from build123d import *

# Parameters (mm, degrees)
BOSS_EXTRUDE1_DEPTH = 5.5
FILLET1_R           = 0.75
FILLET2_R           = 3
SKETCH2_R           = 6
CUT_EXTRUDE1_DEPTH  = 16.19429676984497


with BuildPart() as part:
    # Sketch1 → Boss-Extrude1 (new body)
    with BuildSketch(Plane(origin=(0, 0, 0), x_dir=(1, 0, 0), z_dir=(0, 1, 0))):
        Polygon((10.969655114602853, 0), (5.484827557301405, 9.499999999999982), (-5.48482755730147, 9.499999999999945), (-10.969655114602851, -7.66e-14), (-5.484827557301339, -9.50000000000002), (5.4848275573015375, -9.499999999999904), align=None)
    extrude(amount=BOSS_EXTRUDE1_DEPTH)

    # Fillet1
    fillet1_edges = [part.edges().sort_by_distance(p)[0] for p in [
        (-3.286e-14, 5.5, -9.499999999999964),
        (-8.227241335952161, 5.5, -4.749999999999934),
        (-8.227241335952096, 5.5, 4.750000000000048),
        (9.859e-14, 5.5, 9.499999999999961),
        (8.227241335952195, 5.5, 4.749999999999952),
        (8.22724133595213, 5.5, -4.749999999999991),
    ]]
    fillet(fillet1_edges, radius=FILLET1_R)

    # Fillet2
    # the kernel refuses this fillet: 3 mm, written as the material it takes off along each edge
    with BuildSketch(Plane(origin=(3.752776749732533, 5.5, -6.499999999999977), x_dir=(0.8660254037844382, 0, -0.500000000000001), z_dir=(0.500000000000001, 0, 0.8660254037844382))) as fillet2_piece_1:
        with BuildLine():
            CenterArc((2.25, -0.75), 0.75, 0, 90)
            Line((3, -0.75), (3, 0))
            Line((3, 0), (2.25, 0))
        make_face()
    revolve(axis=Axis((3.752776749732533, 5.5, -6.499999999999977), (0, 1, 0)), revolution_arc=60.000000000000135, mode=Mode.SUBTRACT)
    with BuildSketch(Plane(origin=(7.505553499465103, 5.5, 1.221e-14), x_dir=(0.8660254037844416, 0, 0.49999999999999495), z_dir=(-0.49999999999999495, 0, 0.8660254037844416))) as fillet2_piece_2:
        with BuildLine():
            CenterArc((2.25, -0.75), 0.75, 0, 90)
            Line((3, -0.75), (3, 0))
            Line((3, 0), (2.25, 0))
        make_face()
    revolve(axis=Axis((7.505553499465103, 5.5, 1.221e-14), (0, 1, 0)), revolution_arc=59.99999999999973, mode=Mode.SUBTRACT)
    with BuildSketch(Plane(origin=(-3.752776749732577, 5.5, -6.49999999999995), x_dir=(-3.4e-15, 0, -1), z_dir=(1, 0, -3.4e-15))) as fillet2_piece_3:
        with BuildLine():
            CenterArc((2.25, -0.75), 0.75, 0, 90)
            Line((3, -0.75), (3, 0))
            Line((3, 0), (2.25, 0))
        make_face()
    revolve(axis=Axis((-3.752776749732577, 5.5, -6.49999999999995), (0, 1, 0)), revolution_arc=60.00000000000015, mode=Mode.SUBTRACT)
    with BuildSketch(Plane(origin=(3.7527767497326376, 5.5, 6.499999999999923), x_dir=(1.053e-14, 0, 1), z_dir=(-1, 0, 1.053e-14))) as fillet2_piece_4:
        with BuildLine():
            CenterArc((2.25, -0.75), 0.75, 0, 90)
            Line((3, -0.75), (3, 0))
            Line((3, 0), (2.25, 0))
        make_face()
    revolve(axis=Axis((3.7527767497326376, 5.5, 6.499999999999923), (0, 1, 0)), revolution_arc=59.99999999999973, mode=Mode.SUBTRACT)
    with BuildSketch(Plane(origin=(-7.505553499465096, 5.5, 5.373e-14), x_dir=(-0.8660254037844417, 0, -0.49999999999999484), z_dir=(0.49999999999999484, 0, -0.8660254037844417))) as fillet2_piece_5:
        with BuildLine():
            CenterArc((2.25, -0.75), 0.75, 0, 90)
            Line((3, -0.75), (3, 0))
            Line((3, 0), (2.25, 0))
        make_face()
    revolve(axis=Axis((-7.505553499465096, 5.5, 5.373e-14), (0, 1, 0)), revolution_arc=60.00000000000011, mode=Mode.SUBTRACT)
    with BuildSketch(Plane(origin=(-3.752776749732488, 5.5, 6.500000000000002), x_dir=(-0.8660254037844347, 0, 0.5000000000000068), z_dir=(-0.5000000000000068, 0, -0.8660254037844347))) as fillet2_piece_6:
        with BuildLine():
            CenterArc((2.25, -0.75), 0.75, 0, 90)
            Line((3, -0.75), (3, 0))
            Line((3, 0), (2.25, 0))
        make_face()
    revolve(axis=Axis((-3.752776749732488, 5.5, 6.500000000000002), (0, 1, 0)), revolution_arc=60.00000000000016, mode=Mode.SUBTRACT)
    with BuildSketch(Plane(origin=(-5.484827557301339, -4.330127018922208, 9.50000000000002), x_dir=(1, 0, -1.026e-14), z_dir=(0, 1, 0))) as fillet2_piece_7:
        with BuildLine():
            CenterArc((FILLET2_R * 0.57735026919, FILLET2_R), FILLET2_R, 209.99999999999983, 60.00000000000017)
            Line((-FILLET2_R * 0.288675134595, FILLET2_R * 0.5), (0, 0))
            Line((0, 0), (FILLET2_R * 0.57735026919, 0))
        make_face()
    extrude(amount=9.830127018922209, mode=Mode.SUBTRACT)
    with BuildSketch(Plane(origin=(-10.969655114602851, -4.3301270189222, 7.638e-14), x_dir=(0.4999999999999946, 0, -0.8660254037844417), z_dir=(0, 1, 0))) as fillet2_piece_8:
        with BuildLine():
            CenterArc((FILLET2_R * 0.57735026919, -FILLET2_R), FILLET2_R, 89.99999999999999, 60.00000000000007)
            Line((-FILLET2_R * 0.288675134595, -FILLET2_R * 0.5), (0, 0))
            Line((0, 0), (FILLET2_R * 0.57735026919, 3e-17))
        make_face()
    extrude(amount=9.8301270189222, mode=Mode.SUBTRACT)
    with BuildSketch(Plane(origin=(-5.484827557301471, -4.330127018922209, -9.499999999999945), x_dir=(1, 0, -3.08e-15), z_dir=(0, 1, 0))) as fillet2_piece_9:
        with BuildLine():
            CenterArc((FILLET2_R * 0.57735026919, -FILLET2_R), FILLET2_R, 90.00000000000003, 60.00000000000017)
            Line((-FILLET2_R * 0.288675134595, -FILLET2_R * 0.5), (0, 0))
            Line((0, 0), (FILLET2_R * 0.57735026919, 0))
        make_face()
    extrude(amount=9.830127018922209, mode=Mode.SUBTRACT)
    with BuildSketch(Plane(origin=(5.484827557301404, -4.330127018922204, -9.499999999999982), x_dir=(0.5000000000000011, 0, 0.866025403784438), z_dir=(0, 1, 0))) as fillet2_piece_10:
        with BuildLine():
            CenterArc((FILLET2_R * 0.57735026919, -FILLET2_R), FILLET2_R, 90, 60.00000000000014)
            Line((-FILLET2_R * 0.288675134595, -FILLET2_R * 0.5), (0, 0))
            Line((0, 0), (FILLET2_R * 0.57735026919, 1.1e-16))
        make_face()
    extrude(amount=9.830127018922205, mode=Mode.SUBTRACT)
    with BuildSketch(Plane(origin=(10.969655114602853, -4.330127018922171, 0), x_dir=(-0.500000000000001, 0, -0.8660254037844382), z_dir=(0, 1, 0))) as fillet2_piece_11:
        with BuildLine():
            CenterArc((FILLET2_R * 0.57735026919, FILLET2_R), FILLET2_R, 210.00000000000028, 59.999999999999716)
            Line((-FILLET2_R * 0.288675134595, FILLET2_R * 0.5), (0, 0))
            Line((0, 0), (FILLET2_R * 0.57735026919, 6e-17))
        make_face()
    extrude(amount=9.83012701892217, mode=Mode.SUBTRACT)
    with BuildSketch(Plane(origin=(5.4848275573015375, -4.330127018922169, 9.499999999999904), x_dir=(0.499999999999995, 0, -0.8660254037844415), z_dir=(0, 1, 0))) as fillet2_piece_12:
        with BuildLine():
            CenterArc((FILLET2_R * 0.57735026919, FILLET2_R), FILLET2_R, 210.00000000000028, 59.999999999999716)
            Line((-FILLET2_R * 0.288675134595, FILLET2_R * 0.5), (0, 0))
            Line((0, 0), (FILLET2_R * 0.57735026919, 6e-17))
        make_face()
    extrude(amount=9.83012701892217, mode=Mode.SUBTRACT)

    # Sketch2 → Cut-Extrude1 (cut, through all)
    with BuildSketch(Plane(origin=(0, 5.5, 0), x_dir=(1, 0, 0), z_dir=(0, 1, 0))):
        with Locations(Location((0, 0, 0), (0, 0, 270))):
            Circle(SKETCH2_R)
    extrude(amount=-CUT_EXTRUDE1_DEPTH, mode=Mode.SUBTRACT)


solid = part.part
Source: CAD feature listing. Evaluate the final solid. Frame: model axes, mm. Give positions to 0.01 mm unless a question says otherwise; leave off trailing zeros. Write each loop counter-clockwise with the first axis right and the second up, starting at its lowest first coordinate (ties: lowest second). Pieces come first, ordered by that corner, then holes. Notation, with made-up numbers: (31.25, 80) -> (87.25, 80) arc R19 ccw to (87.25, 93) -> close; hole circle Ø8 at (20.25, 42). An arc over 180 degrees is marked (long way). Return JSON: item names as keys, results as strings. Group by question number.
1. Section A-A, the plane x = 0. Output: boundary loops of the cut face in (y, z).
2. Material intervals for line 1 (X direction, y = 2.55, z = 0); line 2 (X direction, y = 2.5, z = 1.5); line 3 (Z direction, x = -1.5, y = 0.5), sorted ascending. Write a range as from..to.
3. Pin query (flat end, axial travel): pin 1 Ø2 at (y, z) = (2.5, -3) entering from -X; pin 2 Ø2 at (y, z) = (2.5, 7) entering from -X. Return the tip coordinate at first contact, or that it passes through.
4. Mould query, pull axis Z, two halves, no side actions, for faces 1 (the face through (1.802, 2.788, 5.723)), 2 (the face through (-8.07, 5.27, -4.6)), 3 (the face through (-5.27, 2.34, 9.09)). Classes: +Z half, -Z half, draft (parallel to the pull), parting line (faces both ways), or undercut.
5. Section C-C, the plane x = -3.25. Output: boundary loops of the cut face in (y, z).
6. Section B-B, the plane y = 2.6. Output: boundary loops of the cut face in (x, z).
Determined:
{
 "1": {"outline": "(0, -9.5) -> (4.75, -9.5) arc R0.75 ccw to (5.5, -8.75) -> (5.5, -6) -> (0, -6) -> close; (0, 6) -> (5.5, 6) -> (5.5, 8.75) arc R0.75 ccw to (4.75, 9.5) -> (0, 9.5) -> close"},
 "2": {"line 1": "x = -10.51..-6, 6..10.51", "line 2": "x = -10.1..-5.81, 5.81..10.1", "line 3": "z = -9.5..-5.81, 5.81..9.5"},
 "3": {"pin 1": "stops at x = -9.81", "pin 2": "stops at x = -7.51"},
 "4": {"face 1": "undercut", "face 2": "-Z half", "face 3": "+Z half"},
 "5": {"outline": "(0, -9.5) -> (4.75, -9.5) arc R0.75 ccw to (5.5, -8.75) -> (5.5, -5.04) -> (0, -5.04) -> close; (0, 5.04) -> (5.5, 5.04) -> (5.5, 8.75) arc R0.75 ccw to (4.75, 9.5) -> (0, 9.5) -> close"},
 "6": {"outline": "(-10.1, -1.5) -> (-6.35, -8) arc R3 ccw to (-3.75, -9.5) -> (3.75, -9.5) arc R3 ccw to (6.35, -8) -> (10.1, -1.5) arc R3 ccw to (10.1, 1.5) -> (6.35, 8) arc R3 ccw to (3.75, 9.5) -> (-3.75, 9.5) arc R3 ccw to (-6.35, 8) -> (-10.1, 1.5) arc R3 ccw to start; hole circle Ø12 at (0, 0)"}
}
